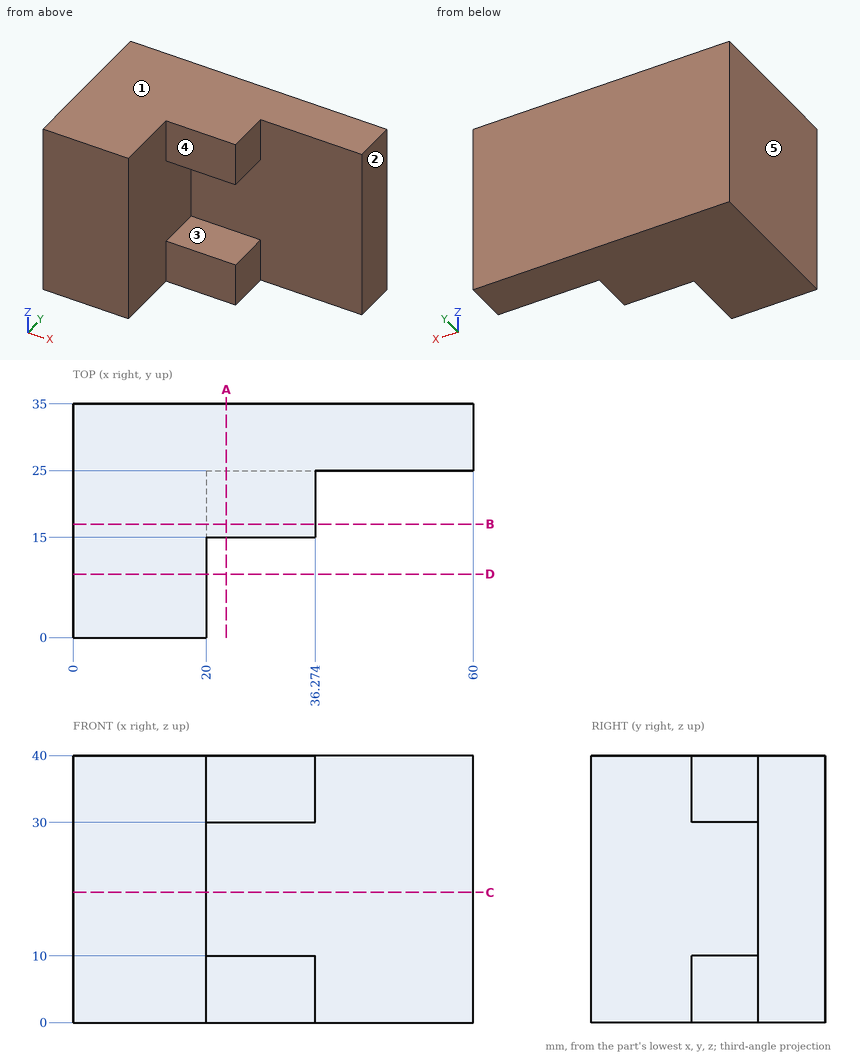
Check sheet for the drawn part. Datum: minimum x, y, z corner. Units: mm. A direction names the side the tool comes from. Round coordinates to 2 decimals unless told otherwise and drop trailing zeros. Loops run counter-clockwise (first coordinate to the right, second up) from the corner with the lowest first, then second, coordinate; pieces in that order, holes last. Notation, with made-up numbers: M -10,84.25 L 26,84.25 A17 ccw 26,110.25 Z; hole C 34.25,50 d4. An arc over 180 degrees is marked long. Write each question's results on one line, items separated by ' | '.
1) Section check A-A on x = 23. Record the boundary of the cut face in (y, z).
Checks:
outline: M 15,0 L 35,0 L 35,40 L 15,40 L 15,30 L 25,30 L 25,10 L 15,10 Z
2) Mould release check, pull along Z, two halves, no side actions. Record for the marked faces 1, 2 and 3: released by +Z, released by -Z, zero draft, split by the parting line, or undercut.
Checks:
face 1: released by +Z | face 2: zero draft | face 3: undercut
3) Access from +Z, -Z, +X, -X, +Y, -Y to the whole of each face (thin tool, end or side, straight path). Record for the marked faces 4 and 5.
Checks:
face 4: +Z, -Z, +X, -Y | face 5: +Z, -Z, -X, +Y, -Y
4) Section check B-B on y = 17. Record the boundary of the cut face in (x, z), then the cut area to 3 significant figures.
Checks:
outline: M 0,0 L 36.27,0 L 36.27,10 L 20,10 L 20,30 L 36.27,30 L 36.27,40 L 0,40 Z | area: 1,130 mm2
5) Section check C-C on z = 19.5. Record the boundary of the cut face in (x, y).
Checks:
outline: M 0,0 L 20,0 L 20,25 L 60,25 L 60,35 L 0,35 Z
6) Gauge pin test, flat ends, axial feed: P1, Ø3, axis at y = 21.5, z = 5, coming from the +X side; P2, Ø12, axis at x = 53.5, z = 19, coming from the -Y side; P3, Ø5, axis at x = 26, z = 33.5, coming from the -Y side. Record the tip position at first contact, or that the pin passes through.
Checks:
P1: stops at x = 36.27 | P2: stops at y = 25 | P3: stops at y = 15
7) Section check D-D on y = 9.5. Record the boundary of the cut face in (x, z).
Checks:
outline: M 0,0 L 20,0 L 20,40 L 0,40 Z
8) Scan lines: L1, parallel to Z at x = 32.5, y = 20.5; L2, parallel to X at y = 4, z = 36; L3, parallel to Y at x = 31, z = 17. Record each from-to range of solid material in increasing order. Write a range as from..to.
Checks:
L1: z = 0..10, 30..40 | L2: x = 0..20 | L3: y = 25..35
